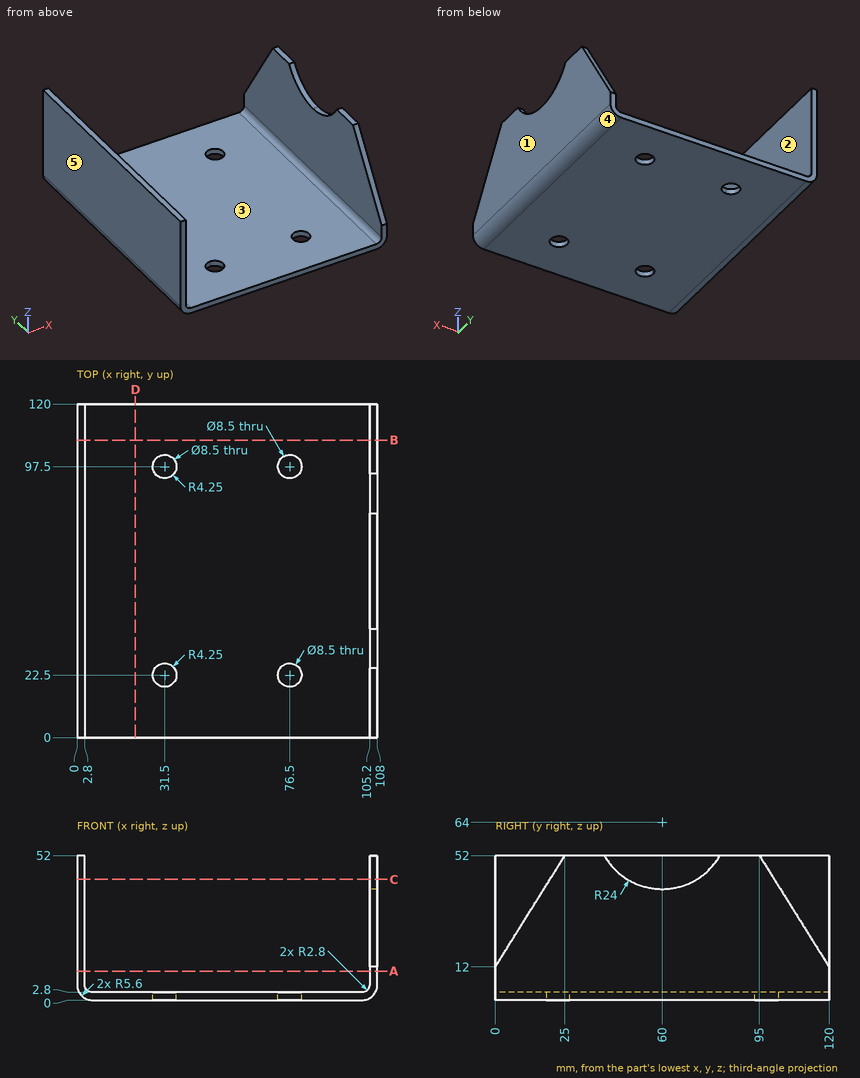
Verification items for this drawing (mm, ordinates from the low corner). A direction names the side the tool comes from. Give positions to 0.01 mm unless a question says otherwise; leave off trailing zeros. Loops run counter-clockwise (first coordinate to the right, second up) from the corner with the lowest first, then second, coordinate; pieces in that order, holes last. Notation, with made-up numbers: M 26,-8 L 83,-8 A21 cw 83,9 Z; hole C -28.75,87 d6. An arc over 180 degrees is marked long. Answer as a JSON object with one key per item and string values. Group by question number.
Item 1: Gauge pin test, flat end, axial feed: pin 1 (10 mm diameter, centred on x = 31.5, y = 97.5, fed in from +Z). Record the tip position at first contact, or that the pin passes through.
Item 2: Sectioned sample at D-D on x = 21. Record the boundary of the cut face in (y, z), plus the area to 3 significant figures.
Item 3: Sectioned sample at A-A on z = 10.5. Record the boundary of the cut face in (x, y), plus the area to 3 significant figures.
Item 4: Sectioned sample at B-B on y = 107. Record the boundary of the cut face in (x, z), plus the area to 3 significant figures.
Item 5: Sectioned sample at C-C on z = 43.5. Record the boundary of the cut face in (x, y), plus the area to 3 significant figures.
Item 6: Mould release check, pull along Z, two halves, no side actions. Record for the marked faces 3, 4 and 5: pulls with the +Z half, pulls with the -Z half, needs draft (parallel to the pull), parting line crosses it, or undercut.
Item 7: Access from +Z, -Z, +X, -X, +Y, -Y to the whole of each face (thin tool, end or side, straight path). Record for the marked faces 1 and 2.
Item 8: Material ranges on L1, parallel to Y at x = 76, z = 2; L2, parallel to X at y = 55.5, z = 27; L3, parallel to X at y = 97.5, z = 2.25, recorded low to high.
Findings below:
{
 "1": {"pin 1": "z = 2.8"},
 "2": {"outline": "M 0,0 L 120,0 L 120,2.8 L 0,2.8 Z", "area": "336 mm2"},
 "3": {"outline": "M 0,0 L 2.8,0 L 2.8,120 L 0,120 Z; M 105.2,0 L 108,0 L 108,120 L 105.2,120 Z", "area": "672 mm2"},
 "4": {"outline": "M 0,5.6 A5.6 ccw 5.6,0 L 102.4,0 A5.6 ccw 108,5.6 L 108,32.8 L 105.2,32.8 L 105.2,5.6 A2.8 cw 102.4,2.8 L 5.6,2.8 A2.8 cw 2.8,5.6 L 2.8,52 L 0,52 Z", "area": "514 mm2"},
 "5": {"outline": "M 0,0 L 2.8,0 L 2.8,120 L 0,120 Z; M 105.2,19.69 L 108,19.69 L 108,47.52 L 105.2,47.52 Z; M 105.2,72.48 L 108,72.48 L 108,100.31 L 105.2,100.31 Z", "area": "492 mm2"},
 "6": {"face 3": "pulls with the +Z half", "face 4": "pulls with the -Z half", "face 5": "needs draft"},
 "7": {"face 1": "+Z, -Z, +X, +Y, -Y", "face 2": "+Z, +Y, -Y"},
 "8": {"L1": "0 to 18.28, 26.72 to 93.28, 101.72 to 120", "L2": "0 to 2.8, 105.2 to 108", "L3": "1.11 to 27.25, 35.75 to 72.25, 80.75 to 106.89"}
}
